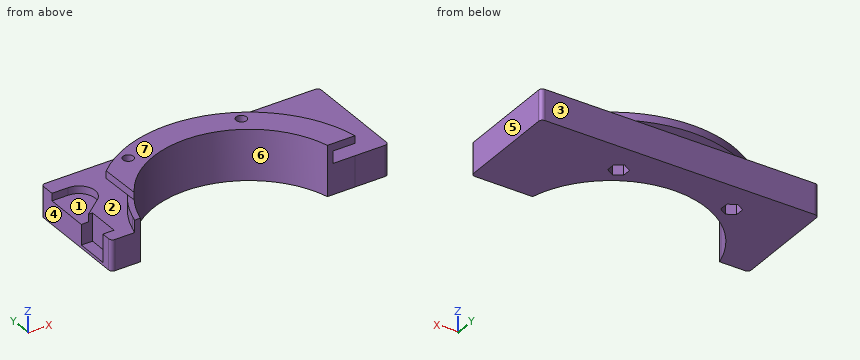
Autodesk Inventor part; units mm, degrees
ref_plane "Work Plane1" through (0, 0, -6.55) normal (0, 0, -1) x (-1, 0, 0)
ref_plane "YZ Plane" through (0, 0, 0) normal (1, 0, 0) x (0, 1, 0)
ref_plane "XZ Plane" through (0, 0, 0) normal (0, 1, 0) x (-1, 0, 0)
sketch "Sketch1" plane through (0, 0, 0) normal (0, 0, 1) x (1, 0, 0)
  arc A0 (162.0167, 39.368) -> (161.237, 51.1295) centre (107.5651, 41.6649) ccw construction
  line L0 (41.1768, 101.6649) -> (144.3643, 101.6649) construction
  circle A1 centre (63.4018, 101.6649) radius 1.75 construction
  line L1 (63.4018, 133.6649) -> (63.4018, 101.6649) construction
  circle A2 centre (107.4018, 101.6649) radius 1.75 construction
  circle A3 centre (151.4018, 101.6649) radius 1.75 construction
  line L2 (151.4018, 133.6649) -> (151.4018, 101.6649) construction
  circle A4 centre (107.5651, 41.6649) radius 50.5415 construction
  line L3 (52.1155, 51.1295) -> (173.6061, 51.1295) construction
  arc A5 (54.2668, 54.0707) -> (55.4284, 57.5398) centre (-8.1112, 76.8868) ccw
  arc A6 (160.627, 54.1023) -> (55.4284, 57.5398) centre (107.5651, 41.6649) ccw
  arc A7 (57.452, 54.0707) -> (58.2983, 56.666) centre (-8.1112, 76.8868) ccw
  arc A8 (157.5424, 54.0957) -> (58.2983, 56.666) centre (107.5651, 41.6649) ccw
  line L4 (172.3778, 54.1273) -> (157.5424, 54.0957)
  line L5 (57.452, 54.0707) -> (43.812, 54.0707)
  arc A9 (172.3778, 54.1273) -> (42.7416, 54.0707) centre (107.5651, 41.6649) ccw
  circle A10 centre (77.3151, 94.0594) radius 2.8
  line L6 (107.5651, 41.6649) -> (77.3151, 94.0594) construction
  line L7 (107.5651, 41.6649) -> (140.5651, 98.8225) construction
  circle A11 centre (137.8151, 94.0594) radius 2.8
  line L8 (63.1685, 103.3992) -> (63.1685, 99.9305)
  line L9 (63.1685, 90.5007) -> (63.5954, 68.4773)
  line L10 (47.625, 54.0707) -> (47.625, 69.2906)
  line L11 (77.1794, 98.965) -> (81.4957, 96.6297)
  line L12 (81.4957, 96.6297) -> (81.7008, 91.6075)
  line L13 (81.7008, 91.6075) -> (77.4508, 89.1538)
  line L14 (77.4508, 89.1538) -> (73.1346, 91.4891)
  line L15 (73.1346, 91.4891) -> (72.9989, 96.3947)
  line L16 (72.9989, 96.3947) -> (77.1794, 98.965)
  line L17 (137.8151, 89.1519) -> (133.5651, 91.6057)
  line L18 (133.5651, 91.6057) -> (133.5651, 96.5131)
  line L19 (133.5651, 96.5131) -> (137.8151, 98.9669)
  line L20 (137.8151, 98.9669) -> (142.0651, 96.5131)
  line L21 (142.0651, 96.5131) -> (142.0651, 91.6057)
  line L22 (142.0651, 91.6057) -> (137.8151, 89.1519)
  line L23 (41.1685, 300.9746) -> (41.1685, 51.9316)
  line L24 (172.3778, 54.1273) -> (188.3778, 54.1273)
  line L25 (172.3778, 54.1273) -> (188.3778, 54.1273) construction
  line L26 (190.3778, 56.1273) -> (190.3778, 108.8269)
  line L27 (188.3778, 110.8269) -> (43.812, 110.8269)
  line L28 (41.812, 56.0707) -> (41.812, 108.8269)
  arc A12 (41.812, 56.0707) -> (43.812, 54.0707) centre (43.812, 56.0707) ccw
  arc A13 (43.812, 110.8269) -> (41.812, 108.8269) centre (43.812, 108.8269) ccw
  arc A14 (190.3778, 108.8269) -> (188.3778, 110.8269) centre (188.3778, 108.8269) ccw
  arc A15 (188.3778, 54.1273) -> (190.3778, 56.1273) centre (188.3778, 56.1273) ccw
  arc A16 (55.9681, 86.6488) -> (50.5185, 102.1453) centre (50.5185, 93.4388) ccw
  line L29 (50.5185, 102.1453) -> (41.812, 102.1453)
  line L30 (41.812, 75.287) -> (55.9681, 86.6488)
  circle A17 centre (50.5185, 93.4388) radius 4.75
  point P0 (0, 0)
  point P1 (107.4018, 133.6649)
  point P2 (190.3778, 54.1273)
  dimension "d18" = 54.5
  dimension "d21" = 3.5
  dimension "d23" = 3.5
  dimension "d24" = 3.5
  dimension "d28" = 60
  dimension "d29" = 3
  dimension "d30" = 5.6
  dimension "d31" = 60.5
  dimension "d32" = 132
  dimension "d33" = 60
  dimension "d34" = 60
  dimension "d35" = 5.6
  dimension "d36" = 60.5
  dimension "d42" = 54.5
  dimension "d49" = 8.5
  dimension "d50" = 8.5
  dimension "d53" = 18
  dimension "d54" = 0
  dimension "d55" = 2
extrude "Extrusion1" add sketch "Sketch1" along normal blind 4 contours L9 A9 L4 A6 | A6 L4 A8 L9 | L11 L12 L13 L14 L15 L16 | L17 L18 L19 L20 L21 L22
extrude "Extrusion2" add sketch "Sketch1" against normal blind 23 contours A5 A6 L9 A8 A7 L5 | A6 L4 A8 L9
ref_plane "Work Plane1" through (0, 0, -6.55) normal (0, 0, -1) x (-1, 0, 0)
extrude "Extrusion3" add sketch "Sketch1" against normal up to surface (16.45 mm away) from surface at -6.55 contours L5 L10 A9 L9 A6 A5 | L5 A12 A9 L10 | L9 A9 L4 A6 | A9 A12 L28 L30 A16 L29 A13 L27 A14 L26 A15 L24 | L28 L29 A16 L30 | L11 L12 L13 L14 L15 L16 | L17 L18 L19 L20 L21 L22 | A17
extrude "Extrusion5" cut sketch "Sketch1" along normal blind 7 from surface at -23 contours L11 L12 L13 L14 L15 L16 | L17 L18 L19 L20 L21 L22
sketch "Sketch3" plane through (41.812, 56.0707, -23) normal (-1, 0, 0) x (0, 0, 1)
  circle A0 centre (7.5, 13.7262) radius 3
  line L0 (16.45, 22.225) -> (1.5875, 22.225)
  line L1 (1.5875, 22.225) -> (1.5875, 4.7625)
  line L2 (1.5875, 4.7625) -> (16.45, 4.7625)
  line L3 (16.45, 4.7625) -> (16.45, 22.225)
  line L4 (16.45, 52.7561) -> (16.45, 0)
  point P0 (23, -56.0707)
extrude "Extrusion6" cut sketch "Sketch3" against normal blind 6 contours A0 | L3 L2 L1 L0
extrude "Extrusion7" cut sketch "Sketch1" against normal blind 4 from surface at -6.55 contours L28 L29 A16 L30 | A17
equation "\"d36\" = d31"
properties part number "Intake Shroud"
Geometry: final body of the model. Coordinates: model frame, mm. Face numbers are marked on the shaded views. A direction names the side the tool comes from. Give positions to 0.01 mm unless a question says otherwise; leave off trailing zeros. Write each loop counter-clockwise with the first axis right and the second up, starting at its lowest first coordinate (ties: lowest second). Pieces come first, ordered by that corner, then holes.
1. Draft query along X for the marked faces 4, 5, 6 and 7. Return one class per face: released by +X, released by -X, zero draft, split by the parting line, or undercut.
2. Section query B-B, the plane z = -4. Return loops of the section in (x, y).
3. Pin query (flat end, axial travel): P1, Ø3, axis at x = 143.5, z = 0, coming from the -Y side; P2, Ø6, axis at x = 144.5, z = 1, coming from the +Y side; P3, Ø4, axis at x = 160, y = 96.5, coming from the +Z side. Return the tip coordinate at first contact, or that it passes through.
4. Section query A-A, the plane y = 105.5. Return loops of the section in (x, z).
5. Section query C-C, the plane z = -12.75. Return loops of the section in (x, y), then the cut area to 3 significant figures.
6. Section query D-D, the plane x = 89.5. Return loops of the section in (y, z), then the cut area to 3 significant figures.
7. Line query: probe 1 along Z at (x, y) = (114, 102); probe 2 along X at (y, z) = (64, -16.5); probe 3 along X at (y, z) = (88, -2.75). Output: solid intervals per line, ascending.
8. Reachability of the marked faces 1, 2 and 3 from +Z, -Z, +X, -X, +Y, -Y: full face, straight path, thin tool, end or side. Return the list, or none.
Computed:
1. face 4: released by -X
1. face 5: released by +X
1. face 6: undercut
1. face 7: zero draft
2. outline: (54.27, 54.07) - (57.45, 54.07) arc R69.32 ccw to (58.3, 56.67) arc R51.5 cw to (157.54, 54.1) - (160.63, 54.1) arc R54.5 ccw to (55.43, 57.54) arc R66.4 cw to start
3. P1: stops at y = 77.03
3. P2: stops at y = 98.27
3. P3: stops at z = -6.55
4. outline: (41.81, -23) - (190.38, -23) - (190.38, -6.55) - (41.81, -6.55) - close; (90.8, 0) - (124.33, 0) - (124.33, 4) - (90.8, 4) - close
5. outline: (41.81, 56.07) arc R2 ccw to (43.81, 54.07) - (57.45, 54.07) arc R69.32 ccw to (58.3, 56.67) arc R51.5 cw to (157.54, 54.1) - (172.38, 54.13) - (188.38, 54.13) arc R2 ccw to (190.38, 56.13) - (190.38, 108.83) arc R2 ccw to (188.38, 110.83) - (43.81, 110.83) arc R2 ccw to (41.81, 108.83) - (41.81, 78.3) - (47.81, 78.3) - (47.81, 60.83) - (41.81, 60.83) - close; hole circle Ø5.6 at (77.32, 94.06); hole circle Ø5.6 at (137.82, 94.06)
5. area: 5,370 mm2
6. outline: (89.89, -23) - (110.83, -23) - (110.83, -6.55) - (93.08, -6.55) - (93.08, 0) - (105.14, 0) - (105.14, 4) - (89.89, 4) - close
6. area: 426 mm2
7. probe 1: z = -23 to -6.55, 0 to 4
7. probe 2: x = 47.81 to 61.16, 153.97 to 190.38
7. probe 3: x = 78.87 to 85.09, 130.04 to 136.26
8. face 1: +Z, -X
8. face 2: +Y
8. face 3: +Z, -Z, +X, -X, +Y
